The listing builds one solid part. Answer for the finished solid, in the listing's coordinates (mm). Face numbers are marked on the shaded views. Round coordinates to 2 decimals unless told otherwise and drop trailing zeros. Write each loop counter-clockwise with the first axis right and the second up, starting at its lowest first coordinate (ties: lowest second). Pieces come first, ordered by that corner, then holes.
Autodesk Inventor part; units mm, degrees
ref_plane "YZ Plane" through (0, 0, 0) normal (1, 0, 0) x (0, 1, 0)
ref_plane "XZ Plane" through (0, 0, 0) normal (0, 1, 0) x (-1, 0, 0)
ref_plane "XY Plane" through (0, 0, 0) normal (0, 0, 1) x (1, 0, 0)
sketch "Эскиз1" plane through (0, 0, 0) normal (0, 0, 1) x (1, 0, 0)
  circle A0 centre (0, 0) radius 13.5 construction
  circle A1 centre (-9.5459, 9.5459) radius 1.25
  line L0 (-9.5459, 9.5459) -> (0, 0) construction
  line L1 (0, 0) -> (2.2284, 0) construction
  circle A2 centre (-9.5459, -9.5459) radius 1.25
  circle A3 centre (9.5459, -9.5459) radius 1.25
  circle A4 centre (9.5459, 9.5459) radius 1.25
  line L2 (17, -17) -> (-17, -17)
  line L3 (-17, -17) -> (-17, 17)
  line L4 (-17, 17) -> (17, 17)
  line L5 (17, 17) -> (17, -17)
  line L6 (17, -17) -> (-17, 17) construction
  line L7 (-17, -17) -> (17, 17) construction
  dimension "d0" = 27
  dimension "d1" = 2.5
  dimension "d3" = 45
  dimension "d6" = 360
  dimension "d8" = 34
  dimension "d9" = 34
extrude "Выдавливание1" add sketch "Эскиз1" along normal blind 10
fillet "Сопряжение1" radius 2 4 edges at (17, 17, 5) (-17, 17, 5) (-17, -17, 5) (17, -17, 5)
sketch "Эскиз2" plane through (-15, 17, 0) normal (0, 1, 0) x (1, 0, 0)
  circle A0 centre (15, -5) radius 1.5
  line L0 (-2, 0) -> (-2, -10)
  line L1 (0, 0) -> (30, 0)
  point P0 (15, 0)
  point P1 (-2, -5)
  point P2 (15, 0)
  dimension "d16" = 3
sketch "Эскиз3" plane through (0, 0, 10) normal (0, 0, 1) x (1, 0, 0)
  circle A0 centre (0, 0) radius 10.1
  dimension "d13" = 20.2
extrude "Выдавливание2" cut sketch "Эскиз3" against normal blind 10
extrude "Выдавливание3" cut sketch "Эскиз2" against normal blind 40.5
chamfer "Фаска1" distance 2 angle 45 5 edges at (-10.7959, 9.5459, 10) (8.2959, 9.5459, 10) (8.2959, -9.5459, 10) (-10.7959, -9.5459, 10) (-1.5, 17, 5)
properties part number "крепление трубы"
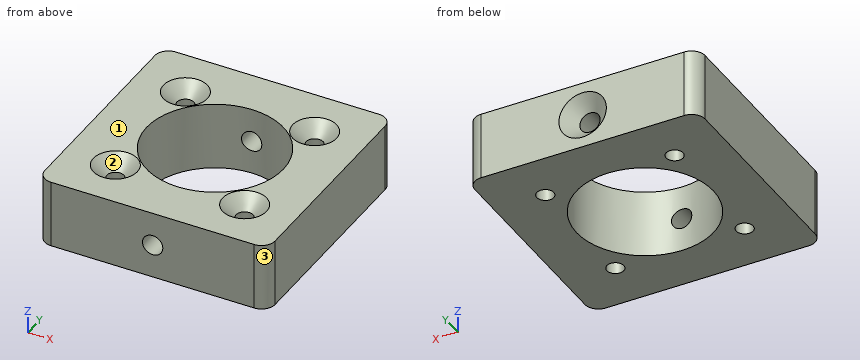
1. Section D-D on z = 2 is taken. Give the number of separate pieces and of enclosed holes in the cut face, plus the area to 3 significant figures.
Geometry says:
separate pieces: 1
enclosed holes: 5
area: 811 mm2
2. Section C-C on z = 5 is taken. Determine the outline of the cut face in (x, y), plus the area to 3 significant figures.
Geometry says:
outline: (-17, -15) arc R2 ccw to (-15, -17) - (-1.5, -17) - (-1.5, -9.99) arc R10.1 cw to (-1.5, 9.99) - (-1.5, 15) - (-3.5, 17) - (-15, 17) arc R2 ccw to (-17, 15) - close; (1.5, -17) - (15, -17) arc R2 ccw to (17, -15) - (17, 15) arc R2 ccw to (15, 17) - (3.5, 17) - (1.5, 15) - (1.5, 9.99) arc R10.1 cw to (1.5, -9.99) - close; hole circle Ø2.5 at (-9.55, -9.55); hole circle Ø2.5 at (-9.55, 9.55); hole circle Ø2.5 at (9.55, -9.55); hole circle Ø2.5 at (9.55, 9.55)
area: 767 mm2
3. Given pin 1 (4 mm diameter, centred on x = 9.55, y = 9.55, fed in from +Z), flat-ended and moving along its own axis, determine where the tip first touches the part or whether it passes through.
Geometry says:
pin 1: stops at z = 8.76
4. Section A-A on y = 0 is taken. Determine the outline of the cut face in (x, z), plus the area to 3 significant figures.
Geometry says:
outline: (-17, 0) - (-10.1, 0) - (-10.1, 10) - (-17, 10) - close; (10.1, 0) - (17, 0) - (17, 10) - (10.1, 10) - close
area: 138 mm2
5. Section B-B on x = 0 is taken. Determine the outline of the cut face in (y, z), plus the area to 3 significant figures.
Geometry says:
outline: (-17, 0) - (-10.1, 0) - (-10.1, 3.5) - (-17, 3.5) - close; (-17, 6.5) - (-10.1, 6.5) - (-10.1, 10) - (-17, 10) - close; (10.1, 0) - (17, 0) - (17, 1.5) - (15, 3.5) - (10.1, 3.5) - close; (10.1, 6.5) - (15, 6.5) - (17, 8.5) - (17, 10) - (10.1, 10) - close
area: 92.6 mm2
6. For a pull along Y with two mould halves and no side action, classify the marked faces 1, 2 and 3 as released by +Y, released by -Y, zero draft, split by the parting line, or undercut.
Geometry says:
face 1: zero draft
face 2: undercut
face 3: released by -Y
7. Straight lines are drawn through the part: line 1 along Z through (x, y) = (0, -14.25); line 2 along Y through (x, z) = (10.5, 1.75); line 3 along Y through (x, z) = (-5, 9). For each, find the intervals that lie inside material, in ascending order.
Geometry says:
line 1: z = 0 to 3.5, 6.5 to 10
line 2: y = -17 to -10.35, -8.74 to 8.74, 10.35 to 17
line 3: y = -17 to -8.78, 8.78 to 17
